Autodesk Inventor part; units mm, degrees
ref_plane "YZ Plane" through (0, 0, 0) normal (1, 0, 0) x (0, 1, 0)
ref_plane "XZ Plane" through (0, 0, 0) normal (0, 1, 0) x (-1, 0, 0)
ref_plane "XY Plane" through (0, 0, 0) normal (0, 0, 1) x (1, 0, 0)
sketch "Sketch1" plane through (0, 0, 0) normal (0, 0, 1) x (1, 0, 0)
  circle A0 centre (0, 0) radius 10
  circle A1 centre (0, 0) radius 20
  line L0 (-15, 0) -> (15, 0)
  line L1 (15, 0) -> (15, 50)
  line L2 (15, 50) -> (-15, 50)
  line L3 (-15, 50) -> (-15, 0)
  point P0 (-15, 13.2288)
  point P1 (15, 13.2288)
  dimension "d0" = 20
  dimension "d1" = 40
  dimension "d2" = 30
  dimension "d3" = 50
extrude "Extrusion1" add sketch "Sketch1" along normal blind 20
sketch "Sketch2" plane through (0, 0, 20) normal (0, 0, 1) x (1, 0, 0)
  circle A0 centre (0, 0) radius 10
  dimension "d6" = 20
extrude "Extrusion2" cut sketch "Sketch2" against normal blind 15
sketch "Sketch3" plane through (0, 0, 20) normal (0, 0, 1) x (1, 0, 0)
  circle A0 centre (0, 0) radius 10
  line L0 (0, 0) -> (6, 0)
  line L1 (6, 0) -> (6, 17)
  line L2 (6, 17) -> (0, 17)
  line L3 (0, 17) -> (0, 0)
  line L4 (0, 0) -> (-6, 0)
  line L5 (-6, 0) -> (-6, 17)
  line L6 (-6, 17) -> (0, 17)
  line L7 (0, 17) -> (0, 0)
  dimension "d9" = 6
  dimension "d10" = 17
  dimension "d11" = 6
  dimension "d12" = 17
sketch "Sketch4" plane through (-15, 13.2288, 0) normal (-1, 0, 0) x (0, 0, 1)
  line L0 (0, 36.7712) -> (20, 36.7712)
  line L1 (0, 0) -> (0, 36.7712)
  line L2 (20, 36.7712) -> (0, 36.7712)
  line L3 (0, 36.7712) -> (0, 0)
  line L4 (0, 0) -> (20, 0)
  line L5 (20, 0) -> (20, 36.7712)
  line L6 (0, 0) -> (20, 0)
  line L7 (20, 36.7712) -> (10, 36.7712)
  line L8 (10, 36.7712) -> (10, 0)
  line L9 (10, 0) -> (20, 0)
  line L10 (20, 0) -> (20, 36.7712)
  line L11 (10, 0) -> (16, 0)
  line L12 (16, 0) -> (16, 25)
  line L13 (16, 25) -> (10, 25)
  line L14 (10, 25) -> (10, 0)
  line L15 (10, 25) -> (4, 25)
  line L16 (4, 25) -> (4, 0)
  line L17 (4, 0) -> (10, 0)
  line L18 (10, 0) -> (10, 25)
  line L19 (4, 25) -> (16, 25)
  line L20 (16, 25) -> (16, 30.0005)
  line L21 (16, 30.0005) -> (4, 30.0005)
  line L22 (4, 30.0005) -> (4, 25)
  line L23 (4, 30.0005) -> (16, 30.0005)
  line L24 (16, 30.0005) -> (16, 7.0005)
  line L25 (16, 7.0005) -> (4, 7.0005)
  line L26 (4, 7.0005) -> (4, 30.0005)
  line L27 (10, 7.0005) -> (16, 7.0005)
  line L28 (16, 7.0005) -> (16, 0)
  line L29 (16, 0) -> (10, 0)
  line L30 (10, 0) -> (10, 7.0005)
  point P0 (0, -13.2288)
  dimension "d13" = 6
  dimension "d14" = 25
  dimension "d15" = 6
  dimension "d16" = 23
extrude "Extrusion3" cut sketch "Sketch4" against normal blind 23 contours L21 L20 L13 L8 | L8 L15 L22 L21 | L13 L12 L25 L8 | L8 L25 L16 L15
sketch "Sketch5" plane through (8, 13.2288, 0) normal (-1, 0, 0) x (0, 0, 1)
  point P0 (0, -13.2288)
sketch "Sketch6" plane through (-15, 13.2288, 0) normal (-1, 0, 0) x (0, 0, 1)
  line L0 (4, 7.0005) -> (4, 30.0005)
  line L1 (4, 7.0005) -> (16, 7.0005)
  line L2 (16, 7.0005) -> (16, 2.2005)
  line L3 (16, 2.2005) -> (4, 2.2005)
  line L4 (4, 2.2005) -> (4, 7.0005)
  line L5 (4, 30.0005) -> (16, 30.0005)
  line L6 (16, 30.0005) -> (16, 34.8005)
  line L7 (16, 34.8005) -> (4, 34.8005)
  line L8 (4, 34.8005) -> (4, 30.0005)
  point P0 (0, -13.2288)
  dimension "d19" = 12
  dimension "d20" = 4.8
  dimension "d21" = 4.8
extrude "Extrusion4" cut sketch "Sketch6" against normal blind 16
sketch "Sketch7" plane through (1, 13.2288, 0) normal (-1, 0, 0) x (0, 0, 1)
  line L0 (4, 30.0005) -> (16, 30.0005)
  line L1 (4, 30.0005) -> (10, 30.0005)
  line L2 (10, 30.0005) -> (10, 32.5005)
  line L3 (10, 32.5005) -> (4, 32.5005)
  line L4 (4, 32.5005) -> (4, 30.0005)
  circle A0 centre (10, 32.5005) radius 0.75
  line L5 (16, 7.0005) -> (4, 7.0005)
  line L6 (16, 7.0005) -> (16, 2.2005)
  line L7 (4, 7.0005) -> (16, 7.0005)
  line L8 (16, 7.0005) -> (16, 4.5005)
  line L9 (16, 4.5005) -> (4, 4.5005)
  line L10 (4, 4.5005) -> (4, 7.0005)
  line L11 (10, 4.5005) -> (4, 4.5005)
  line L12 (4, 4.5005) -> (4, 7.0005)
  line L13 (4, 7.0005) -> (10, 7.0005)
  line L14 (10, 7.0005) -> (10, 4.5005)
  circle A1 centre (10, 4.5005) radius 0.75
  point P0 (0, -13.2288)
  dimension "d24" = 2.5
  dimension "d25" = 1.5
  dimension "d26" = 2.5
  dimension "d27" = 1.5
extrude "Extrusion5" cut sketch "Sketch7" against normal blind 8 contours A0 L3 L2 | L2 L3 A0 | A1 L9 L14 | L14 L9 A1 | A1 L9
sketch "Sketch8" plane through (15, 13.2288, 0) normal (1, 0, 0) x (0, 0, -1)
  line L0 (0, 36.7712) -> (0, 0)
  line L1 (-20, 36.7712) -> (-20, 0)
  line L2 (0, 36.7712) -> (-20, 36.7712)
  line L3 (-20, 36.7712) -> (-20, 26.7712)
  line L4 (-20, 26.7712) -> (0, 26.7712)
  line L5 (0, 26.7712) -> (0, 36.7712)
  line L6 (0, 26.7712) -> (-20, 26.7712)
  line L7 (-20, 26.7712) -> (-20, 18.7712)
  line L8 (-20, 18.7712) -> (0, 18.7712)
  line L9 (0, 18.7712) -> (0, 26.7712)
  line L10 (0, 26.7712) -> (-10, 26.7712)
  line L11 (-10, 26.7712) -> (-10, 18.7712)
  line L12 (-10, 18.7712) -> (0, 18.7712)
  line L13 (0, 18.7712) -> (0, 26.7712)
  line L14 (-10, 26.7712) -> (-5, 26.7712)
  line L15 (-5, 26.7712) -> (-5, 22.7712)
  line L16 (-5, 22.7712) -> (-10, 22.7712)
  line L17 (-10, 22.7712) -> (-10, 26.7712)
  line L18 (-10, 22.7712) -> (-15, 22.7712)
  line L19 (-15, 22.7712) -> (-15, 26.7712)
  line L20 (-15, 26.7712) -> (-10, 26.7712)
  line L21 (-10, 26.7712) -> (-10, 22.7712)
  point P0 (0, -13.2288)
  dimension "d30" = 10
  dimension "d31" = 8
  dimension "d32" = 5
  dimension "d33" = 5
extrude "Extrusion6" cut sketch "Sketch8" against normal blind 15.8125 contours L15 L16 L11 L4 | L11 L18 L19 L4
sketch "Sketch9" plane through (0, 0, 5) normal (0, 0, 1) x (1, 0, 0)
  circle A0 centre (0, 0) radius 1
  circle A1 centre (7, 0) radius 1.5
  circle A2 centre (0, 0) radius 1.5
  circle A3 centre (-7, 0) radius 1.5
  dimension "d36" = 2
  dimension "d37" = 3
  dimension "d38" = 3
  dimension "d39" = 3
extrude "Extrusion7" cut sketch "Sketch9" against normal blind 8 contours A0 | A1 | A2 | A3
chamfer "Chamfer1" distance 8 angle 45 1 edges at (-10, 0, 20)
properties part number "EndConnector"
Here's how the part is built. I have some questions about the finished solid (model axes, mm). A direction names the side the tool comes from. Round coordinates to 2 decimals unless told otherwise and drop trailing zeros. Loops run counter-clockwise (first coordinate to the right, second up) from the corner with the lowest first, then second, coordinate; pieces in that order, holes last. Notation, with made-up numbers: (-32, -15) -> (24, -15) arc R15 cw to (24, 8) -> close; hole circle Ø2 at (43, -27.75). An arc over 180 degrees is marked (long way). Answer as CSV lines item,"result".
1. If we section it at C-C on y = 39: Please give me the cut outline in (x, z).
Final values:
outline,"(-15, 0) -> (15, 0) -> (15, 5) -> (8, 5) -> (8, 4) -> (-15, 4) -> close; (-15, 16) -> (8, 16) -> (8, 15) -> (15, 15) -> (15, 20) -> (-15, 20) -> close"
2. Which directions (+Z, -Z, +X, -X, +Y, -Y) give clear straight access to the entire face, cutting with the end or side of a thin tool? Please do faces 1 (the face through (12, 36, 10)), 2 (the face through (-2.17, -9.76, 8.55)), 3 (the face through (1, 44.6, 9.9)), 4 (the face through (15, 31, 10)).
Final values:
face 1,"+X, -X"
face 2,"+Z"
face 3,"-X"
face 4,"+Z, -Z, +X, +Y"
3. If we section it at A-A on z = 10: Please give me the cut outline in (x, y).
Final values:
outline,"(-15, 13.23) arc R20 ccw (long way) to (15, 13.23) -> (15, 36) -> (8, 36) -> (8, 20.23) -> (1, 20.23) -> (1, 18.48) -> (9, 18.48) -> (9, 16.98) -> (1, 16.98) -> (1, 15.43) -> (-15, 15.43) -> close; (-15, 48.03) -> (1, 48.03) -> (1, 46.48) -> (9, 46.48) -> (9, 44.98) -> (1, 44.98) -> (1, 43.23) -> (8, 43.23) -> (8, 40) -> (15, 40) -> (15, 50) -> (-15, 50) -> close; hole circle Ø20 at (0, 0)"
4. If we section it at B-B on x = 0: Please give me the cut outline in (y, z).
Final values:
outline,"(-20, 0) -> (-1.5, 0) -> (-1.5, 5) -> (-10, 5) -> (-10, 12) -> (-18, 20) -> (-20, 20) -> close; (1.5, 0) -> (50, 0) -> (50, 20) -> (18, 20) -> (10, 12) -> (10, 5) -> (1.5, 5) -> close; hole (15.43, 4) -> (48.03, 4) -> (48.03, 16) -> (15.43, 16) -> close"
5. For pin 1 (4 mm diameter, centred on y = 19.5, z = 4.5, fed in from +X); pin 2 (3.5 mm diameter, centred on x = 12, z = 7.5, fed in from -Y); pin 3 (2 mm diameter, centred on y = -3, z = 3, fed in from -X), each with a flat end and sliding along its axis, tell me the tip position at first contact or that it passes through.
Final values:
pin 1,"stops at x = 15"
pin 2,"stops at y = -17.17"
pin 3,"stops at x = -19.9"
6. Thinking about a two-plate mould opening in Y: for faces 5 (the face through (0, 50, 10)), 6 (the face through (8, 29, 10)), 7 (the face through (-7, 48.029, 10)), 8 (the face through (0, 15, 0)), which applies, released by +Y, released by -Y, zero draft, split by the parting line, or undercut?
Final values:
face 5,"released by +Y"
face 6,"undercut"
face 7,"undercut"
face 8,"zero draft"
7. If I drill on L1, parallel to Y at x = 0, z = 9.75; L2, parallel to Y at x = 4, z = 13.5; L3, parallel to Z at x = 6.5, y = 43, over which ranges is the centre line in solid material (lowest first)?
Final values:
L1,"y = -20 to -10, 10 to 15.43, 48.03 to 50"
L2,"y = -19.6 to -10.78, 10.78 to 20.23, 43.23 to 50"
L3,"z = 0 to 4, 16 to 20"
8. If we section it at D-D on z = 1.75: Please give me the cut outline in (x, y).
Final values:
outline,"(-15, 13.23) arc R20 ccw (long way) to (15, 13.23) -> (15, 50) -> (-15, 50) -> close; hole circle Ø3 at (-7, 0); hole circle Ø3 at (0, 0); hole circle Ø3 at (7, 0)"
